Input: dimensioned drawing with shaded views. Units: mm. Origin: part minimum x, y, z. A direction names the side the tool comes from. Give positions to 0.01 mm unless a question says otherwise; leave off trailing zeros. Loops run counter-clockwise (first coordinate to the right, second up) from the corner with the lowest first, then second, coordinate; pieces in that order, holes last.
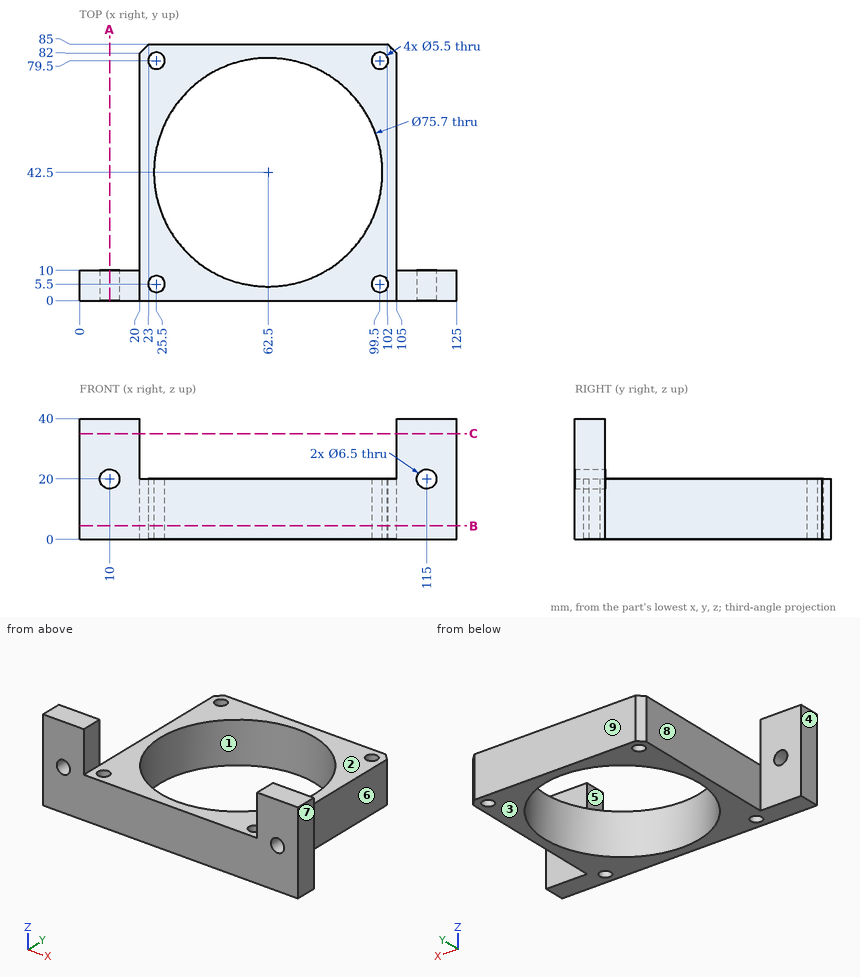
(1) Mould query, pull axis X, two halves, no side actions, for the marked faces 1, 2, 3 and 4. Classes: pulls with the +X half, pulls with the -X half, needs draft (parallel to the pull), parting line crosses it, or undercut.
A:
face 1: undercut
face 2: undercut
face 3: needs draft
face 4: pulls with the -X half
(2) Reachability of the marked faces 5, 6, 7, 8 and 9 from +Z, -Z, +X, -X, +Y, -Y: full face, straight path, thin tool, end or side. Return the list, or none.
A:
face 5: +Z, +Y, -Y
face 6: +Z, -Z, +X, +Y
face 7: +Z, -Z, +X, +Y, -Y
face 8: +Z, -Z, -X, +Y
face 9: +Z, -Z, +X, -X, +Y
(3) Ray query, line 1 along Z through (x, y) = (10, 3.5); line 2 along Z through (x, y) = (22.5, 37); line 3 along Y through (x, z) = (9, 26). Return the intervals inside material, ascending.
A:
line 1: z = 0 to 16.75, 23.25 to 40
line 2: z = 0 to 20
line 3: y = 0 to 10
(4) Section C-C, the plane z = 35. Return the cut outline in (x, y), then the cut area to 3 significant figures.
A:
outline: (0, 0) - (20, 0) - (20, 10) - (0, 10) - close; (105, 0) - (125, 0) - (125, 10) - (105, 10) - close
area: 400 mm2
(5) First-contact query: pin 1 (1 mm diameter, centred on y = 26.5, z = 21.5, fed in from -X); pin 2 (16 mm diameter, centred on y = 52.5, z = 12.5, fed in from -X); pin 3 (6 mm diameter, centred on x = 120, z = 21.5, fed in from +Y); pin 4 (1 mm diameter, centred on x = 100.5, y = 64, fed in from +Z). Flat tips, straight axial feed; report the tip coordinate or a pass-through.
A:
pin 1: passes through
pin 2: stops at x = 20
pin 3: stops at y = 10
pin 4: stops at z = 20
(6) Section A-A, the plane x = 10. Return the cut outline in (y, z).
A:
outline: (0, 0) - (10, 0) - (10, 16.75) - (0, 16.75) - close; (0, 23.25) - (10, 23.25) - (10, 40) - (0, 40) - close
(7) Section B-B, the plane z = 4.5. Return the cut outline in (x, y).
A:
outline: (0, 0) - (125, 0) - (125, 10) - (105, 10) - (105, 82) - (102, 85) - (23, 85) - (20, 82) - (20, 10) - (0, 10) - close; hole circle Ø5.5 at (25.5, 5.5); hole circle Ø5.5 at (25.5, 79.5); hole circle Ø75.7 at (62.5, 42.5); hole circle Ø5.5 at (99.5, 5.5); hole circle Ø5.5 at (99.5, 79.5)
